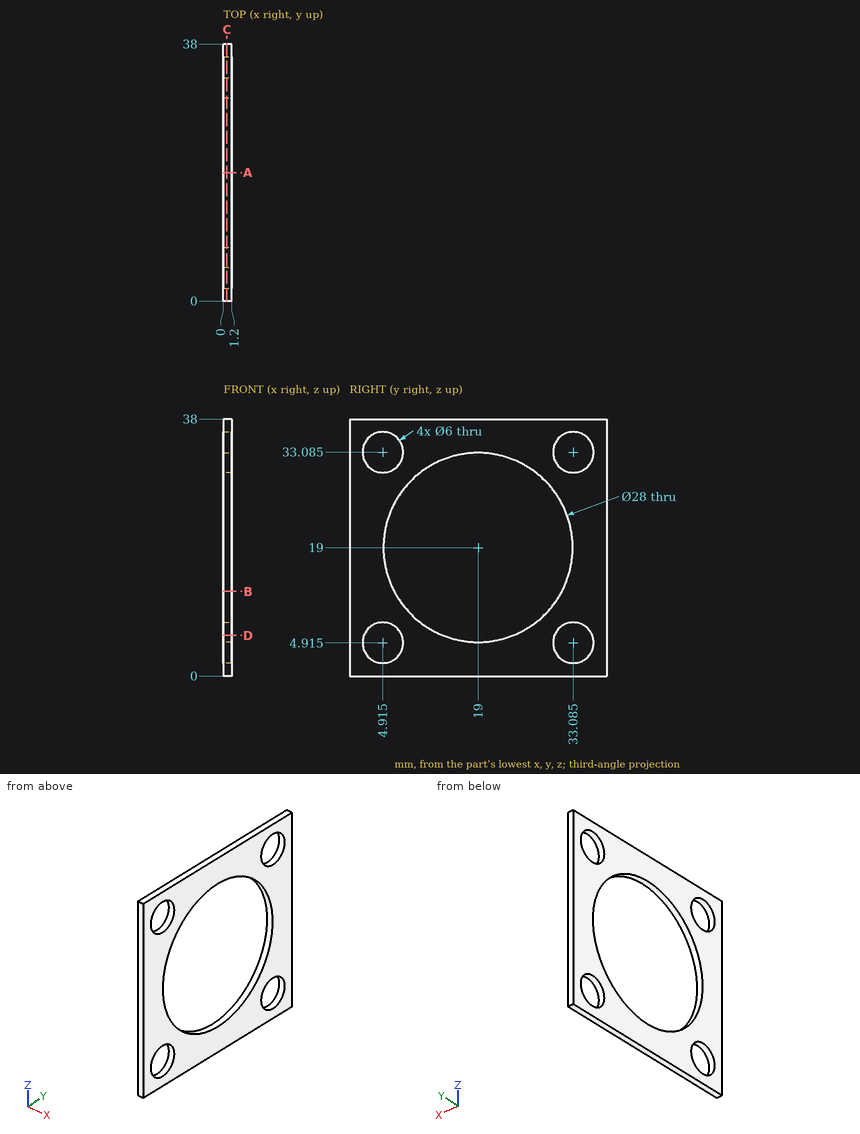
Check sheet for the drawn part. Datum: minimum x, y, z corner. Units: mm. Give positions to 0.01 mm unless a question says otherwise; leave off trailing zeros. Order: outer loops, then holes, each group sorted by start corner. A loop starts at its lowest first (then second) coordinate and runs counter-clockwise, first axis right, second up.
1. Sectioned sample at B-B (z = 12.5). Record the boundary of the cut face in (x, y), then the cut area to 3 significant figures.
Completed:
outline: (0, 0) - (1.2, 0) - (1.2, 6.6) - (0, 6.6) - close; (0, 31.4) - (1.2, 31.4) - (1.2, 38) - (0, 38) - close
area: 15.8 mm2
2. Sectioned sample at A-A (y = 19). Record the boundary of the cut face in (x, z), then the cut area to 3 significant figures.
Completed:
outline: (0, 0) - (1.2, 0) - (1.2, 5) - (0, 5) - close; (0, 33) - (1.2, 33) - (1.2, 38) - (0, 38) - close
area: 12.0 mm2
3. Depth check by flat-ended pin: pin 1 (5 mm diameter, centred on y = 4.915, z = 33.085, fed in from +X). Enter the tip coordinate at first touch or a pass-through.
Completed:
pin 1: passes through
4. Scan lines: line 1 (Y direction, x = 0.6, z = 19.5); line 2 (Y direction, x = 0.5, z = 7); line 3 (Z direction, x = 1.1, y = 35). Record each from-to range of solid material in increasing order.
Completed:
line 1: y = 0 to 5.01, 32.99 to 38
line 2: y = 0 to 2.76, 7.07 to 11.79, 26.21 to 30.93, 35.24 to 38
line 3: z = 0 to 2.61, 7.22 to 30.78, 35.39 to 38
5. Sectioned sample at C-C (x = 0.5). Record the boundary of the cut face in (y, z) (3 decimals), then the cut area to 3 significant figures.
Completed:
outline: (0, 0) - (38, 0) - (38, 38) - (0, 38) - close; hole circle Ø6 at (4.915, 4.915); hole circle Ø6 at (4.915, 33.085); hole circle Ø28 at (19, 19); hole circle Ø6 at (33.085, 4.915); hole circle Ø6 at (33.085, 33.085)
area: 715 mm2
6. Sectioned sample at D-D (z = 6). Record the boundary of the cut face in (x, y), then the cut area to 3 significant figures.
Completed:
outline: (0, 0) - (1.2, 0) - (1.2, 2.12) - (0, 2.12) - close; (0, 7.71) - (1.2, 7.71) - (1.2, 13.8) - (0, 13.8) - close; (0, 24.2) - (1.2, 24.2) - (1.2, 30.29) - (0, 30.29) - close; (0, 35.88) - (1.2, 35.88) - (1.2, 38) - (0, 38) - close
area: 19.7 mm2
